```python
from build123d import *

# Parameters (mm, degrees)
SKICA1_R                 = 2.5
P_IDAT_VYSUNUT_M1_DEPTH  = 8
SKICA2_R                 = 3.75
P_IDAT_VYSUNUT_M2_DEPTH  = 6.25
ODEBRAT_VYSUNUT_M1_DEPTH = 3.75
ZKOSEN_1_SIZE            = 0.25


with BuildPart() as part:
    # Skica1 → Přidat vysunutím1 (new body)
    with BuildSketch(Plane(origin=(0, 0, 0), x_dir=(1, 0, 0), z_dir=(0, 1, 0))):
        with Locations(Location((0, 0, 0), (0, 0, 270))):
            Circle(SKICA1_R)
    extrude(amount=P_IDAT_VYSUNUT_M1_DEPTH)

    # Skica2 → Přidat vysunutím2 (add)
    with BuildSketch(Plane(origin=(0, 8, 0), x_dir=(1, 0, 0), z_dir=(0, 1, 0))):
        with Locations(Location((0, 0, 0), (0, 0, 270))):
            Circle(SKICA2_R)
    extrude(amount=P_IDAT_VYSUNUT_M2_DEPTH)

    # Skica3 → Odebrat vysunutím1 (cut)
    with BuildSketch(Plane(origin=(0, 14.25, 0), x_dir=(1, 0, 0), z_dir=(0, 1, 0))):
        Polygon((-0.199101745, -2.300802431), (1.893002482, -1.322828385), (2.092104227, 0.977974047), (0.199101745, 2.300802431), (-1.893002482, 1.322828385), (-2.092104227, -0.977974047), align=None)
    extrude(amount=-ODEBRAT_VYSUNUT_M1_DEPTH, mode=Mode.SUBTRACT)

    # Zkosení1
    zkosen_1_edges = [part.edges().sort_by_distance(p)[0] for p in [
        (0, 0, -2.5),
        (0, 14.25, -3.75),
    ]]
    chamfer(zkosen_1_edges, length=ZKOSEN_1_SIZE)


solid = part.part
```
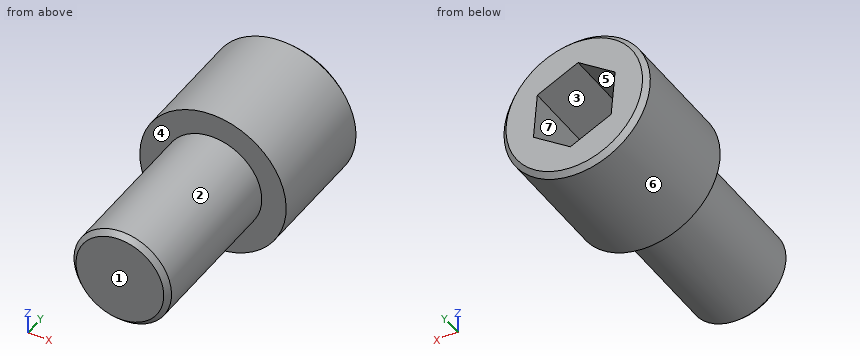
Build history of the part. All positions in model axes, mm. Face numbers are marked on the shaded views. A direction names the side the tool comes from. Round coordinates to 2 decimals unless told otherwise and drop trailing zeros. Order: outer loops, then holes, each group sorted by start corner. A loop starts at its lowest first (then second) coordinate and runs counter-clockwise, first axis right, second up. Notation, with made-up numbers: (-4, 26) - (24, 26) arc R16 cw to (24, 38) - close; hole circle Ø9 at (4.5, 39). An arc over 180 degrees is marked (long way). Use a Markdown table: item, result.
1) Tool access for the marked faces 1, 2 and 3: list every direction of +Z, -Z, +X, -X, +Y, -Y with a clear straight run to the whole face (end or side of a thin tool).
Recorded:
| item | result |
|---|---|
| face 1 | +Z, -Z, +X, -X, -Y |
| face 2 | -Y |
| face 3 | +Y |
2) Pull direction Z, two halves, no side cores. Call the marked faces 4, 5, 6 and 7: pulls with the +Z half, pulls with the -Z half, needs draft (parallel to the pull), parting line crosses it, or undercut.
Recorded:
| item | result |
|---|---|
| face 4 | needs draft |
| face 5 | undercut |
| face 6 | parting line crosses it |
| face 7 | undercut |
3) Saw through at B-B on y = 5. Write the cut outline in (x, z).
Recorded:
| item | result |
|---|---|
| outline | circle Ø5 at (0, 0) |
4) Saw through at C-C on x = 0. Write the cut outline in (y, z), and give its area (3 significant figures).
Recorded:
| item | result |
|---|---|
| outline | (0, -2.25) - (0.25, -2.5) - (8, -2.5) - (8, -3.75) - (14, -3.75) - (14.25, -3.5) - (14.25, -2.21) - (10.5, -2.21) - (10.5, 2.21) - (14.25, 2.21) - (14.25, 3.5) - (14, 3.75) - (8, 3.75) - (8, 2.5) - (0.25, 2.5) - (0, 2.25) - close |
| area | 70.2 mm² |
5) Flat gauge pins, fed straight in: pin 1 Ø1.5 at (x, y) = (0, 6.5) entering from +Z; pin 2 Ø3 at (y, z) = (6, -2.5) entering from +X. Where does each tip first touch, or does it go through?
Recorded:
| item | result |
|---|---|
| pin 1 | stops at z = 2.5 |
| pin 2 | stops at x = 2.29 |
6) Saw through at A-A on z = 0. Write the cut outline in (x, y), and give its area (3 significant figures).
Recorded:
| item | result |
|---|---|
| outline | (-3.75, 8) - (-2.5, 8) - (-2.5, 0.25) - (-2.25, 0) - (2.25, 0) - (2.5, 0.25) - (2.5, 8) - (3.75, 8) - (3.75, 14) - (3.5, 14.25) - (2.01, 14.25) - (2.01, 10.5) - (-2.01, 10.5) - (-2.01, 14.25) - (-3.5, 14.25) - (-3.75, 14) - close |
| area | 71.7 mm² |
7) Wall check: L1, parallel to Y at x = 3, z = -0.75; L2, parallel to Z at x = 3, y = 12; L3, parallel to X at y = 13, z = -1.25. Give the ranges that are in metal, low to high.
Recorded:
| item | result |
|---|---|
| L1 | y = 8 to 14.25 |
| L2 | z = -2.25 to 2.25 |
| L3 | x = -3.54 to -1.9, 1.7 to 3.54 |
